Geometry: final body of the model. Coordinates: model frame, mm. Face numbers are marked on the shaded views. Round coordinates to 2 decimals unless told otherwise and drop trailing zeros. Loops run counter-clockwise (first coordinate to the right, second up) from the corner with the lowest first, then second, coordinate; pieces in that order, holes last. Notation, with made-up numbers: (86.25, 24.25) -> (125.25, 24.25) arc R30 cw to (125.25, 62.25) -> close; hole circle Ø5 at (49.5, 26.5). An arc over 180 degrees is marked (long way). Answer in a Markdown table with one row per item.
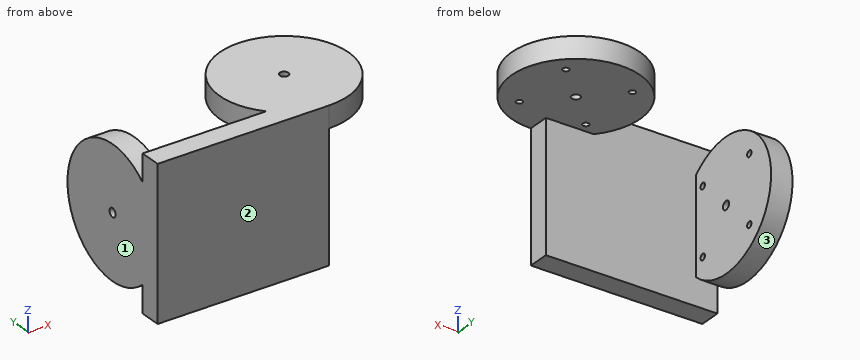
```python
from build123d import *

# Parameters (mm, degrees)
SKETCH1_R                   = 30
BOSS_EXTRUDE1_DEPTH         = 10
SKETCH2_W                   = 80
SKETCH2_H                   = 10
BOSS_EXTRUDE2_DEPTH         = 70
SKETCH3_R                   = 30
BOSS_EXTRUDE3_DEPTH         = 10
F_4_0MM_DOWEL_HOLE1_D       = 4
F_4_0MM_DOWEL_HOLE1_DEPTH   = 10.1
F_4_0MM_DOWEL_HOLE1_TIP     = 1.201721238
M3_5X0_6_TAPPED_HOLE1_D     = 2.9
M3_5X0_6_TAPPED_HOLE1_DEPTH = 8.8
M3_5X0_6_TAPPED_HOLE1_TIP   = 0.871247898
F_4_0MM_DOWEL_HOLE5_D       = 4
F_4_0MM_DOWEL_HOLE5_DEPTH   = 10.1
F_4_0MM_DOWEL_HOLE5_TIP     = 1.201721238
M3_5X0_6_TAPPED_HOLE4_D     = 2.9
M3_5X0_6_TAPPED_HOLE4_DEPTH = 8.8
M3_5X0_6_TAPPED_HOLE4_TIP   = 0.871247898


with BuildPart() as part:
    # Sketch1 → Boss-Extrude1 (new body)
    with BuildSketch(Plane.XY):
        Circle(SKETCH1_R)
    extrude(amount=BOSS_EXTRUDE1_DEPTH)

    # Sketch2 → Boss-Extrude2 (add)
    with BuildSketch(Plane.XY.offset(10)):
        with Locations((-40, -25)):
            Rectangle(SKETCH2_W, SKETCH2_H)
    extrude(amount=-BOSS_EXTRUDE2_DEPTH)

    # Sketch3 → Boss-Extrude3 (add)
    with BuildSketch(Plane.ZY.offset(80)):
        with Locations((-25, 0)):
            Circle(SKETCH3_R)
    extrude(amount=-BOSS_EXTRUDE3_DEPTH)

    # Ø4.0mm Dowel Hole1
    with Locations(Plane(origin=(0, 0, 0), x_dir=(-1, 0, 0), z_dir=(0, 0, -1))):
        with Locations((0, 0)):
            Hole(F_4_0MM_DOWEL_HOLE1_D / 2, depth=F_4_0MM_DOWEL_HOLE1_DEPTH)
            with Locations((0, 0, -(F_4_0MM_DOWEL_HOLE1_DEPTH + F_4_0MM_DOWEL_HOLE1_TIP / 2))):  # 118° drill point
                Cone(0, F_4_0MM_DOWEL_HOLE1_D / 2, F_4_0MM_DOWEL_HOLE1_TIP, mode=Mode.SUBTRACT)

    # M3.5x0.6 Tapped Hole1
    with Locations(Plane(origin=(0, 0, 0), x_dir=(-1, 0, 0), z_dir=(0, 0, -1))):
        with Locations((-15.5, 15.5), (15.5, 15.5), (15.5, -15.5), (-15.5, -15.5)):
            Hole(M3_5X0_6_TAPPED_HOLE1_D / 2, depth=M3_5X0_6_TAPPED_HOLE1_DEPTH)
            with Locations((0, 0, -(M3_5X0_6_TAPPED_HOLE1_DEPTH + M3_5X0_6_TAPPED_HOLE1_TIP / 2))):  # 118° drill point
                Cone(0, M3_5X0_6_TAPPED_HOLE1_D / 2, M3_5X0_6_TAPPED_HOLE1_TIP, mode=Mode.SUBTRACT)

    # Ø4.0mm Dowel Hole5
    with Locations(Plane(origin=(-70, 13.498610341, 45.984792648), x_dir=(0, 0, -1), z_dir=(1, 0, 0))):
        with Locations((70.984792648, -13.498610341)):
            Hole(F_4_0MM_DOWEL_HOLE5_D / 2, depth=F_4_0MM_DOWEL_HOLE5_DEPTH)
            with Locations((0, 0, -(F_4_0MM_DOWEL_HOLE5_DEPTH + F_4_0MM_DOWEL_HOLE5_TIP / 2))):  # 118° drill point
                Cone(0, F_4_0MM_DOWEL_HOLE5_D / 2, F_4_0MM_DOWEL_HOLE5_TIP, mode=Mode.SUBTRACT)

    # M3.5x0.6 Tapped Hole4
    with Locations(Plane(origin=(-70, 0.743323111, -25.05678535), x_dir=(0, 0, -1), z_dir=(1, 0, 0))):
        with Locations((-15.55678535, 14.756676889), (15.44321465, 14.756676889), (15.44321465, -16.243323111), (-15.55678535, -16.243323111)):
            Hole(M3_5X0_6_TAPPED_HOLE4_D / 2, depth=M3_5X0_6_TAPPED_HOLE4_DEPTH)
            with Locations((0, 0, -(M3_5X0_6_TAPPED_HOLE4_DEPTH + M3_5X0_6_TAPPED_HOLE4_TIP / 2))):  # 118° drill point
                Cone(0, M3_5X0_6_TAPPED_HOLE4_D / 2, M3_5X0_6_TAPPED_HOLE4_TIP, mode=Mode.SUBTRACT)


solid = part.part
```
Item 1: Section query C-C, the plane x = -73. Output: boundary loops of the cut face in (y, z), and give its area (3 significant figures).
Ans:
| item | result |
|---|---|
| outline | (-30, -60) -> (-20, -60) -> (-20, -47.36) arc R30 ccw (long way) to (-20, -2.64) -> (-20, 10) -> (-30, 10) -> close; hole circle Ø2.9 at (-15.5, -40.5); hole circle Ø2.9 at (-15.5, -9.5); hole circle Ø4 at (0, -25); hole circle Ø2.9 at (15.5, -40.5); hole circle Ø2.9 at (15.5, -9.5) |
| area | 3,180 mm2 |
Item 2: Section query B-B, the plane y = -12.5. Output: boundary loops of the cut face in (x, z).
Ans:
| item | result |
|---|---|
| outline | (-80, -52.27) -> (-70, -52.27) -> (-70, 2.27) -> (-80, 2.27) -> close; (-27.27, 0) -> (27.27, 0) -> (27.27, 10) -> (-27.27, 10) -> close |
Item 3: Mould query, pull axis Y, two halves, no side actions, for the marked faces 1, 2 and 3. Classes: released by +Y, released by -Y, zero draft, split by the parting line, or undercut.
Ans:
| item | result |
|---|---|
| face 1 | zero draft |
| face 2 | released by -Y |
| face 3 | undercut |
Item 4: First-contact query: P1, Ø5, axis at x = -18.5, z = -10.5, coming from the +Y side; P2, Ø2.5, axis at y = -15.5, z = -40.5, coming from the +X side; P3, Ø2.5, axis at x = -15.5, y = -15.5, coming from the -Z side; P4, Ø18, axis at x = -8, y = -13.5, coming from the -Z side. Flat tips, straight axial feed; report the tip coordinate or a pass-through.
Ans:
| item | result |
|---|---|
| P1 | y = -20 |
| P2 | x = -78.92 |
| P3 | z = 8.92 |
| P4 | z = -60 |
Item 5: Section query D-D, the plane x = -59. Output: boundary loops of the cut face in (y, z).
Ans:
| item | result |
|---|---|
| outline | (-30, -60) -> (-20, -60) -> (-20, 10) -> (-30, 10) -> close |
Item 6: Section query A-A, the plane y = 0. Output: boundary loops of the cut face in (x, z), and give its area (3 significant figures).
Ans:
| item | result |
|---|---|
| outline | (-80, -55) -> (-70, -55) -> (-70, -27) -> (-80, -27) -> close; (-80, -23) -> (-70, -23) -> (-70, 5) -> (-80, 5) -> close; (-30, 0) -> (-2, 0) -> (-2, 10) -> (-30, 10) -> close; (2, 0) -> (30, 0) -> (30, 10) -> (2, 10) -> close |
| area | 1,120 mm2 |
Item 7: Ray query, L1, parallel to Y at x = -75.5, z = -40.5; L2, parallel to Y at x = -75, z = -40; L3, parallel to X at y = 11, z = -9. Return the intervals inside material, ascending.
Ans:
| item | result |
|---|---|
| L1 | -30 to -16.95, -14.05 to 14.05, 16.95 to 25.69 |
| L2 | -30 to -16.86, -14.14 to 14.14, 16.86 to 25.98 |
| L3 | -80 to -70 |
